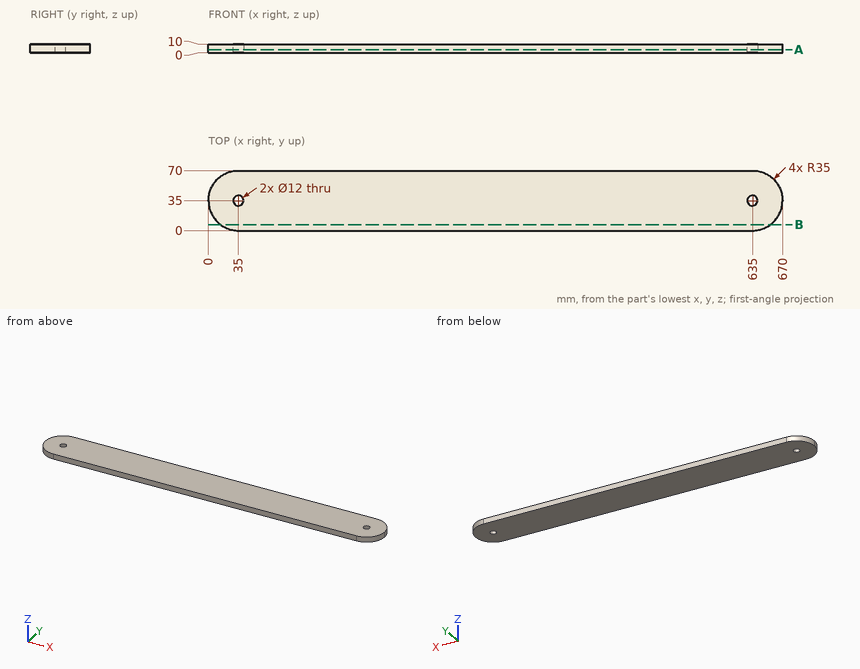
Print and shaded views of the part. All mm, measured from the part's lowest x, y and z. Give positions to 0.01 mm unless a question says otherwise; leave off trailing zeros. Loops run counter-clockwise (first coordinate to the right, second up) from the corner with the lowest first, then second, coordinate; pieces in that order, holes last. Notation, with made-up numbers: (-13, 4) -> (22, 4) arc R12 ccw to (22, 18) -> close; hole circle Ø5 at (32.5, 84.5). An arc over 180 degrees is marked (long way). Use CSV: the item, a comma, the result in double quotes. Start each with the question number.
1) Wall check: line 1 (Y direction, x = 635, z = 4.25); line 2 (X direction, y = 6, z = 0.75); line 3 (X direction, y = 11, z = 4.75) (1 decimal). Give the ranges that are in metal, low to high.
2) Slice it at B-B on y = 7. Give the cut face in (x, z), plus the area to 3 significant figures.
3) Flat gauge pins, fed straight in: pin 1 Ø1.5 at (x, z) = (257, 5.5) entering from -Y; pin 2 Ø1.5 at (y, z) = (13, 9) entering from -X; pin 3 Ø3 at (y, z) = (21.5, 2) entering from +X. Where does each tip first touch, or does it go through?
4) Slice it at A-A on z = 3.5. Give the number of separate pieces and of enclosed holes in the cut face, plus the area to 3 significant figures.
Computed values:
1,line 1,"y = 0 to 29, 41 to 70"
1,line 2,"x = 15.4 to 654.6"
1,line 3,"x = 9.5 to 660.5"
2,outline,"(14, 0) -> (656, 0) -> (656, 10) -> (14, 10) -> close"
2,area,"6,420 mm^2"
3,pin 1,"stops at y = 0"
3,pin 2,"stops at x = 7.19"
3,pin 3,"stops at x = 667.88"
4,separate pieces,"1"
4,enclosed holes,"2"
4,area,"45,600 mm^2"
